Check sheet for the modelled part. Datum: model origin and axes. Units: mm. A direction names the side the tool comes from. Give positions to 0.01 mm unless a question says otherwise; leave off trailing zeros. Order: outer loops, then holes, each group sorted by start corner. A loop starts at its lowest first (then second) coordinate and runs counter-clockwise, first axis right, second up. Notation, with made-up numbers: (53, 6) -> (92, 6) arc R24 ccw to (92, 17) -> close; hole circle Ø5 at (2, 18). An arc over 180 degrees is marked (long way). Answer in a Markdown table with one row per item. Add a question column.
(1) Go/stop test with flat-tipped pins: pin 1 (4 mm diameter, centred on x = 12, z = 5, fed in from -Y); pin 2 (8 mm diameter, centred on y = 24.5, z = 10, fed in from -X); pin 3 (6 mm diameter, centred on x = 9.5, y = -5.5, fed in from +Z). Record where each tip stops, or that it passes through.
(2) Release check for a two-part mould opening along Y. For faces 3 (the face through (-4.101, 31.232, 2.958)), 4 (the face through (-5.961, -26.846, 15.86)), 5 (the face through (-28.1, 9.5, 6)) record: released by +Y, released by -Y, zero draft, split by the parting line, or undercut.
(3) Cross-section at C-C (z = 21.25). Record the cut outline in (x, y), then the cut area to 3 significant figures.
(4) Cross-section at D-D (z = 4.5). Record the cut outline in (x, y).
(5) Thickness scan on L1, parallel to Y at x = 0, z = 13.5; L2, parallel to Z at x = 13, y = 3; L3, parallel to Y at x = 6.5, z = 6.25. Record the ranges inside material, lowest first. Write a range as [from, to].
(6) Set-up check for faces 1 (the face through (0, 0, 0)), 2 (the face through (28.14, 8.86, 14.87)): record each of +Z, -Z, +X, -X, +Y, -Y from which the full face is reachable in a straight line by a thin tool's end or side.
```python
from build123d import *

# Parameters (mm, degrees)
ESBO_O1_R                = 31.5
RESSALTO_EXTRUS_O1_DEPTH = 6
ESBO_O2_R                = 29.5
ESBO_O2_R_2              = 27.5
RESSALTO_EXTRUS_O2_DEPTH = 20
CHANFRO1_SIZE            = 2


with BuildPart() as part:
    # Esboço1 → Ressalto-extrusão1 (new body)
    with BuildSketch(Plane.XY):
        Circle(ESBO_O1_R)
    extrude(amount=RESSALTO_EXTRUS_O1_DEPTH)

    # Esboço2 → Ressalto-extrusão2 (add)
    with BuildSketch(Plane.XY.offset(6)):
        Circle(ESBO_O2_R)
        Circle(ESBO_O2_R_2, mode=Mode.SUBTRACT)
    extrude(amount=RESSALTO_EXTRUS_O2_DEPTH)

    # Chanfro1
    chanfro1_edges = [part.edges().sort_by_distance(p)[0] for p in [
        (-29.5, 0, 26),
    ]]
    chamfer(chanfro1_edges, length=CHANFRO1_SIZE - 0.0001)  # a hair under: the kernel refuses the full size


solid = part.part
```
Answer below:
| question | item | result |
|---|---|---|
| 1 | pin 1 | stops at y = -29.87 |
| 1 | pin 2 | stops at x = -21.21 |
| 1 | pin 3 | stops at z = 6 |
| 2 | face 3 | split by the parting line |
| 2 | face 4 | undercut |
| 2 | face 5 | zero draft |
| 3 | outline | circle Ø59 at (0, 0); hole circle Ø55 at (0, 0) |
| 3 | area | 358 mm² |
| 4 | outline | circle Ø63 at (0, 0) |
| 5 | L1 | y = [-29.5, -27.5], [27.5, 29.5] |
| 5 | L2 | z = [0, 6] |
| 5 | L3 | y = [-28.77, -26.72], [26.72, 28.77] |
| 6 | face 1 | -Z, +X, -X, +Y, -Y |
| 6 | face 2 | +Z |
